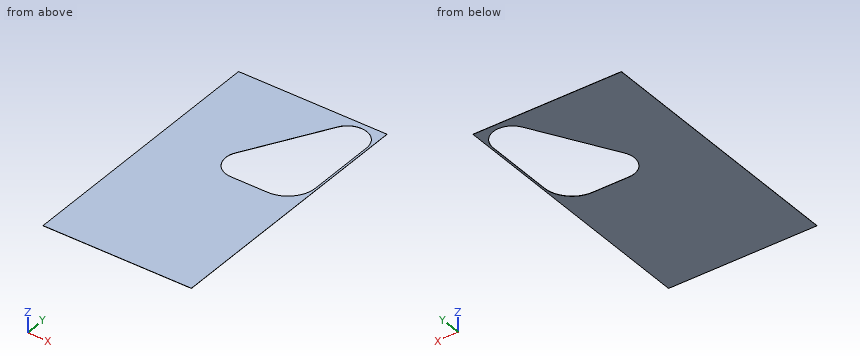
from build123d import *

# Parameters (mm, degrees)
SKETCH1_W           = 903
SKETCH1_H           = 1625
BOSS_EXTRUDE1_DEPTH = 1
CUT_EXTRUDE1_DEPTH  = 1957.486620094


with BuildPart() as part:
    # Sketch1 → Boss-Extrude1 (new body)
    with BuildSketch(Plane.XY):
        with Locations((451.5, 812.5)):
            Rectangle(SKETCH1_W, SKETCH1_H)
    extrude(amount=BOSS_EXTRUDE1_DEPTH)

    # Sketch2 → Cut-Extrude1 (cut, through all)
    with BuildSketch(Plane(origin=(-119.436638294, -43.071405931, 1), x_dir=(1, 0, 0), z_dir=(0, 0, 1))):
        with BuildLine():
            Line((1010.436638294, 1516.071405931), (1010.436638294, 1091.071405931))
            ThreePointArc((1010.436638294, 1091.071405931), (961.230577533, 972.277466691), (842.436638294, 923.071405931))
            Line((842.436638294, 923.071405931), (618.195260429, 923.071405931))
            ThreePointArc((618.195260429, 923.071405931), (516.004262782, 982.071405931), (516.004262782, 1100.071405931))
            Line((516.004262782, 1100.071405931), (790.245640647, 1575.071405931))
            ThreePointArc((790.245640647, 1575.071405931), (922.977285616, 1630.050653433), (1010.436638294, 1516.071405931))
        make_face()
    extrude(amount=-CUT_EXTRUDE1_DEPTH, mode=Mode.SUBTRACT)


solid = part.part
The listing builds one solid part. Answer for the finished solid, in the listing's coordinates (mm). Give positions to 0.01 mm unless a question says otherwise; leave off trailing zeros. Write each loop counter-clockwise with the first axis right and the second up, starting at its lowest first coordinate (ties: lowest second). Pieces come first, ordered by that corner, then holes. Notation, with made-up numbers: (3.25, -5.5) -> (60.25, -5.5) arc R12 ccw to (60.25, 7.5) -> close; hole circle Ø7 at (71.5, 35). An arc over 180 degrees is marked (long way). Use a Markdown table: item, result.
(1) Section C-C, the plane x = 442.5 is taken. Determine the outline of the cut face in (y, z), then the cut area to 3 significant figures.
Return value:
| item | result |
|---|---|
| outline | (0, 0) -> (894.27, 0) -> (894.27, 1) -> (0, 1) -> close; (1136.56, 0) -> (1625, 0) -> (1625, 1) -> (1136.56, 1) -> close |
| area | 1,380 mm2 |
(2) Section A-A, the plane z = 0.2 is taken. Determine the outline of the cut face in (x, y), then the cut area to 3 significant figures.
Return value:
| item | result |
|---|---|
| outline | (0, 0) -> (903, 0) -> (903, 1625) -> (0, 1625) -> close; hole (396.57, 1057) arc R118 ccw to (498.76, 880) -> (723, 880) arc R168 ccw to (891, 1048) -> (891, 1473) arc R118 ccw to (670.81, 1532) -> close |
| area | 1,210,000 mm2 |
(3) Section B-B, the plane y = 989 is taken. Determine the outline of the cut face in (x, z).
Return value:
| item | result |
|---|---|
| outline | (0, 0) -> (381.1, 0) -> (381.1, 1) -> (0, 1) -> close; (880.3, 0) -> (903, 0) -> (903, 1) -> (880.3, 1) -> close |
(4) Find the intervals of material crossed by probe 1 along Y at (x, z) = (671, 0.8); probe 2 along X at (y, z) = (1444, 0.55); probe 3 along X at (y, z) = (974.5, 0.35), in increasing order. Write a range as from..to.
Return value:
| item | result |
|---|---|
| probe 1 | 0..880, 1532.33..1625 |
| probe 2 | 0..620, 891..903 |
| probe 3 | 0..383.12, 874.07..903 |
